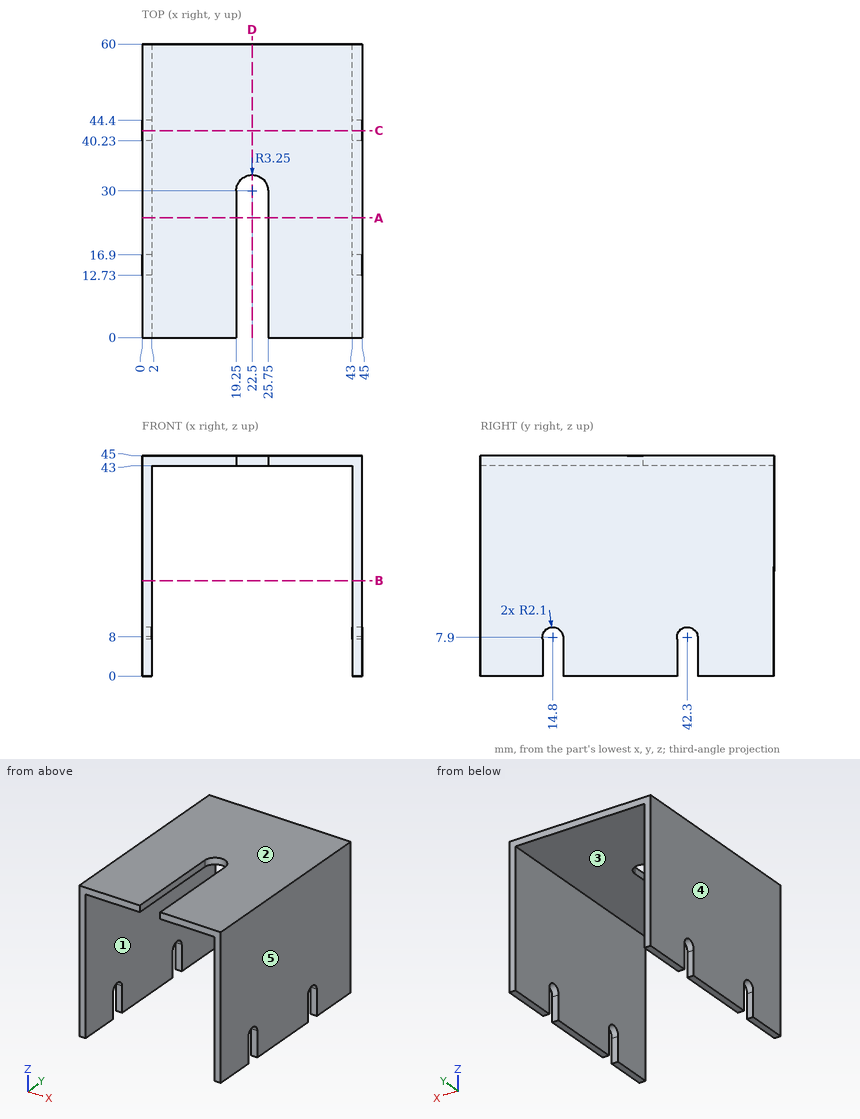
Design review of the part shown in the three views and the two pictorial views. Dimensions are in mm from the part's minimum x, y and z. A direction names the side the tool comes from. Round coordinates to 2 decimals unless told otherwise and drop trailing zeros. Loops run counter-clockwise (first coordinate to the right, second up) from the corner with the lowest first, then second, coordinate; pieces in that order, holes last.
Q1. Add section D-D on x = 22.5. Write out the cut boundary in (y, z), plus the area to 3 significant figures.
Result sheet:
outline: (33.25, 43) - (60, 43) - (60, 45) - (33.25, 45) - close
area: 53.5 mm2
Q2. Add section B-B on z = 19.5. Write out the cut boundary in (x, y), plus the area to 3 significant figures.
Result sheet:
outline: (0, 0) - (2, 0) - (2, 60) - (0, 60) - close; (43, 0) - (45, 0) - (45, 60) - (43, 60) - close
area: 240 mm2
Q3. Mouldability with a two-part tool opening along X and no side actions: class the marked faces 3, 4 and 5 as +X half, -X half, draft (parallel to the pull), parting line (faces both ways), or undercut.
Result sheet:
face 3: undercut
face 4: -X half
face 5: +X half
Q4. To check wall thickness, follow line 1 along X through (y, z) = (20, 43.5); line 2 along X through (y, z) = (11, 12); line 3 along Z through (x, y) = (14, 42.5). State the ranges of each line that lie inside material, in increasing order.
Result sheet:
line 1: x = 0 to 19.25, 25.75 to 45
line 2: x = 0 to 2, 43 to 45
line 3: z = 43 to 45
Q5. Add section A-A on y = 24.5. Write out the cut boundary in (x, z), plus the area to 3 significant figures.
Result sheet:
outline: (0, 0) - (2, 0) - (2, 43) - (19.25, 43) - (19.25, 45) - (0, 45) - close; (25.75, 43) - (43, 43) - (43, 0) - (45, 0) - (45, 45) - (25.75, 45) - close
area: 249 mm2
Q6. Machinability: for the marked faces 1 and 2, which of the approach directions +Z, -Z, +X, -X, +Y, -Y give a long, thin tool a straight path to every point of the face, cutting with its end or side? Answer none if there is none.
Result sheet:
face 1: -Z, +Y, -Y
face 2: +Z, +X, -X, +Y, -Y
Q7. Add section C-C on y = 42.3. Write out the cut boundary in (x, z).
Result sheet:
outline: (0, 10) - (2, 10) - (2, 43) - (43, 43) - (43, 10) - (45, 10) - (45, 45) - (0, 45) - close
Q8. Insertion check: pin 1 Ø12 at (x, z) = (13, 9) entering from -Y; pin 2 Ø12.5 at (x, y) = (23, 31.5) entering from -Z. Each pin has a flat end and moves straight along its axis. Give the tip position at first contact, or say it passes through.
Result sheet:
pin 1: passes through
pin 2: stops at z = 43
